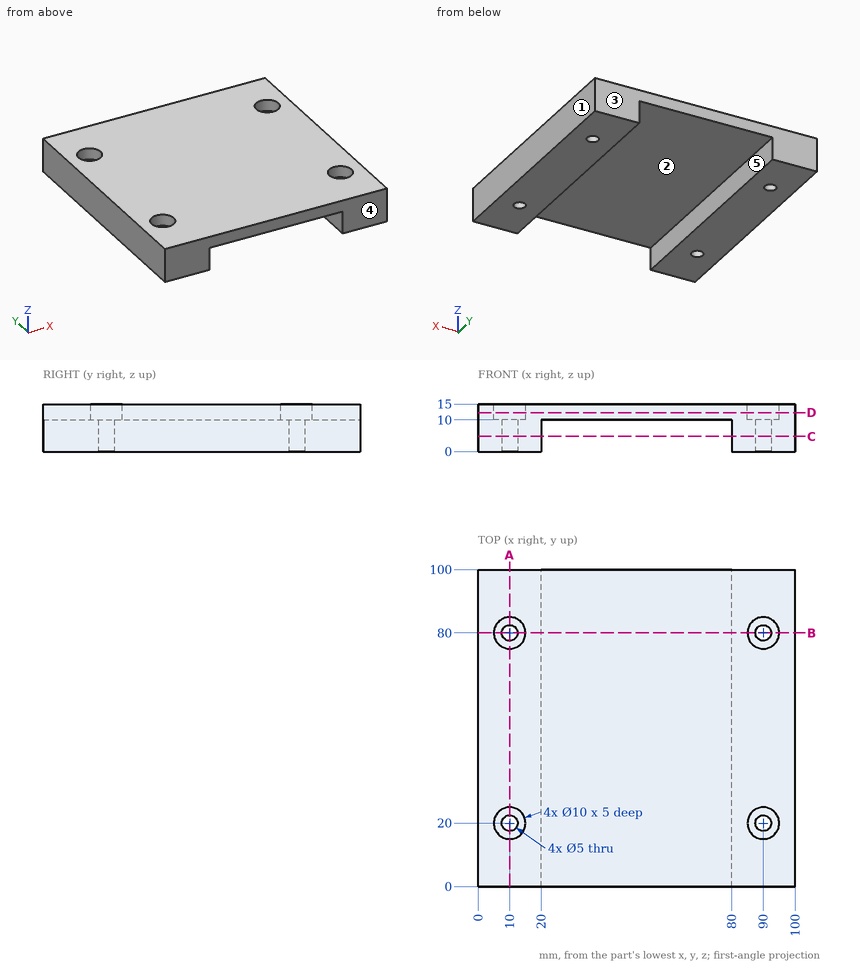
Design review of the part shown in the three views and the two pictorial views. Dimensions are in mm from the part's minimum x, y and z. A direction names the side the tool comes from. Round coordinates to 2 decimals unless told otherwise and drop trailing zeros. Loops run counter-clockwise (first coordinate to the right, second up) from the corner with the lowest first, then second, coordinate; pieces in that order, holes last. Notation, with made-up numbers: M 43,-3.5 L 48,-3.5 A14 ccw 48,6.5 Z; hole C 21.25,38 d11. An arc over 180 degrees is marked long. Write item = value, one per line.
Item 1: Take a section at A-A on x = 10. Write out the cut boundary in (y, z), then the cut area to 3 significant figures.
Return value:
outline = M 0,0 L 17.5,0 L 17.5,10 L 15,10 L 15,15 L 0,15 Z; M 22.5,0 L 77.5,0 L 77.5,10 L 75,10 L 75,15 L 25,15 L 25,10 L 22.5,10 Z; M 82.5,0 L 100,0 L 100,15 L 85,15 L 85,10 L 82.5,10 Z
area = 1,300 mm2
Item 2: Take a section at C-C on z = 4.75. Write out the cut boundary in (x, y), then the cut area to 3 significant figures.
Return value:
outline = M 0,0 L 20,0 L 20,100 L 0,100 Z; M 80,0 L 100,0 L 100,100 L 80,100 Z; hole C 10,20 d5; hole C 10,80 d5; hole C 90,20 d5; hole C 90,80 d5
area = 3,920 mm2
Item 3: For line 1 (Y direction, x = 90, z = 11.2); line 2 (X direction, y = 48, z = 9.5); line 3 (X direction, y = 80, z = 2.25), list the stretches that pass through material, from the lowest coordinate up. Write a range as [from, to].
Return value:
line_1 = [0, 15], [25, 75], [85, 100]
line_2 = [0, 20], [80, 100]
line_3 = [0, 7.5], [12.5, 20], [80, 87.5], [92.5, 100]
Item 4: Insertion check: P1, Ø18, axis at x = 35.5, y = 40, coming from the -Z side; P2, Ø3, axis at x = 90, y = 81.5, coming from the +Z side. Each pin has a flat end and moves straight along its axis. Give the tip position at first contact, or say it passes through.
Return value:
P1 = 10
P2 = 10
Item 5: Machinability: for the marked faces 4 and 5, which of the approach directions +Z, -Z, +X, -X, +Y, -Y give a long, thin tool a straight path to every point of the face, cutting with its end or side? Answer none if there is none.
Return value:
face_4 = +Z, -Z, +X, -X, -Y
face_5 = -Z, +Y, -Y
Item 6: The part is to be moulded in two halves that separate along X. For the marked faces 1, 2 and 3, say which applies: released by +X, released by -X, zero draft, split by the parting line, or undercut.
Return value:
face_1 = released by +X
face_2 = undercut
face_3 = zero draft
Item 7: Take a section at B-B on y = 80. Write out the cut boundary in (x, z).
Return value:
outline = M 0,0 L 7.5,0 L 7.5,10 L 5,10 L 5,15 L 0,15 Z; M 12.5,0 L 20,0 L 20,10 L 80,10 L 80,0 L 87.5,0 L 87.5,10 L 85,10 L 85,15 L 15,15 L 15,10 L 12.5,10 Z; M 92.5,0 L 100,0 L 100,15 L 95,15 L 95,10 L 92.5,10 Z
Item 8: Take a section at D-D on z = 12.25. Write out the cut boundary in (x, y), then the cut area to 3 significant figures.
Return value:
outline = M 0,0 L 100,0 L 100,100 L 0,100 Z; hole C 10,20 d10; hole C 10,80 d10; hole C 90,20 d10; hole C 90,80 d10
area = 9,690 mm2
